Verification items for the finished model (mm, model axes). A direction names the side the tool comes from. Give positions to 0.01 mm unless a question says otherwise; leave off trailing zeros. Loops run counter-clockwise (first coordinate to the right, second up) from the corner with the lowest first, then second, coordinate; pieces in that order, holes last. Notation, with made-up numbers: (-37.75, 2.5) - (10.25, 2.5) arc R15 ccw to (10.25, 14.5) - close; hole circle Ø11 at (-4, -37.5). An arc over 180 degrees is marked (long way). Use one line per item in the form item = value.
```python
from build123d import *

# Parameters (mm, degrees)
EXTRUDE_1_DEPTH     = 5
SKETCH_2_R          = 1.5
CUT_EXTRUDE_1_DEPTH = 318


with BuildPart() as part:
    # 草图1 → 凸台-拉伸1 (new body)
    with BuildSketch(Plane.XY):
        Polygon((78, 5.370967742), (76.5, 5.370967742), (76.5, 0.870967742), (-76.5, 0.870967742), (-76.5, 5.370967742), (-78, 5.370967742), (-78, 0.629032258), (-78, -0.629032258), (78, -0.629032258), (78, 0.629032258), align=None)
    extrude(amount=EXTRUDE_1_DEPTH)

    # 草图2 → 切除-拉伸1 (cut)
    with BuildSketch(Plane.ZY.offset(78)):
        with Locations((2.5, 2.970967742)):
            Circle(SKETCH_2_R)
    extrude(amount=-CUT_EXTRUDE_1_DEPTH, mode=Mode.SUBTRACT)


solid = part.part
```
1. Scan lines: probe 1 along Y at (x, z) = (-77.6, 2.5); probe 2 along X at (y, z) = (1.1, 0.5); probe 3 along Y at (x, z) = (-47, 4.6). Record each from-to range of solid material in increasing order.
Result set:
probe_1 = -0.63 to 1.47, 4.47 to 5.37
probe_2 = -78 to -76.5, 76.5 to 78
probe_3 = -0.63 to 0.87
2. Draft check along Y on faces 3 (the flat face through (-1, -0.629, 2)), 4 (the flat face through (-78, 1, 2)), 5 (the cylindrical face through (77.239, 4.458, 2.305)). Enter one of: released by +Y, released by -Y, zero draft, split by the parting line, or undercut.
Result set:
face_3 = released by -Y
face_4 = zero draft
face_5 = undercut
3. Tool access check on faces 1 (the flat face through (1, 0.871, 2)), 2 (the flat face through (78, 1, 2)). Record the directions out of +Z, -Z, +X, -X, +Y, -Y that give a thin tool (end or side, any length) a straight path to the whole face; none if there is none.
Result set:
face_1 = +Z, -Z, +Y
face_2 = +Z, -Z, +X, +Y, -Y
4. Section check B-B, the plane x = 56. Record the cut outline in (y, z).
Result set:
outline = (-0.63, 0) - (0.87, 0) - (0.87, 5) - (-0.63, 5) - close
5. Section check A-A, the plane z = 2.5. Record the cut outline in (x, y).
Result set:
outline = (-78, -0.63) - (78, -0.63) - (78, 1.47) - (76.5, 1.47) - (76.5, 0.87) - (-76.5, 0.87) - (-76.5, 1.47) - (-78, 1.47) - close; (-78, 4.47) - (-76.5, 4.47) - (-76.5, 5.37) - (-78, 5.37) - close; (76.5, 4.47) - (78, 4.47) - (78, 5.37) - (76.5, 5.37) - close
6. Depth check by flat-ended pin: pin 1 Ø2.5 at (x, z) = (-15, 2.5) entering from +Y. Enter the tip coordinate at first touch or a pass-through.
Result set:
pin_1 = 0.87
